Design review of the part built by this model. Coordinates are the model's own, in mm. Face numbers are marked on the shaded views. A direction names the side the tool comes from. Give positions to 0.01 mm unless a question says otherwise; leave off trailing zeros. Loops run counter-clockwise (first coordinate to the right, second up) from the corner with the lowest first, then second, coordinate; pieces in that order, holes last. Notation, with made-up numbers: (79, 87) -> (114, 87) arc R8 cw to (114, 94) -> close; hole circle Ø5 at (2.25, 1.25). An arc over 180 degrees is marked (long way). Answer as CSV lines item,"result".
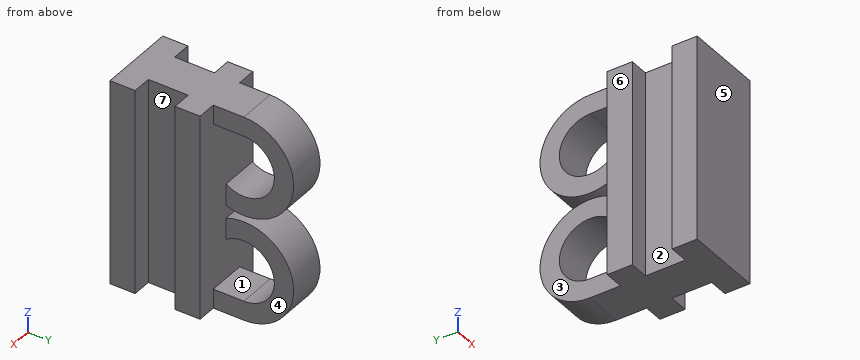
from build123d import *

# Parameters (mm, degrees)
SKETCH1_W           = 15.995688374
SKETCH1_H           = 2
SKETCH1_H_2         = 3
BOSS_EXTRUDE1_DEPTH = 3
SKETCH4_W           = 15.995688374
SKETCH4_H           = 1.95
BOSS_EXTRUDE2_DEPTH = 3


with BuildPart() as part:
    # Sketch1 → Boss-Extrude1 (new body)
    with BuildSketch(Plane(origin=(0, 0, 0), x_dir=(0, 0, -1), z_dir=(1, 0, 0))):
        with BuildLine():
            Line((-7.997844187, 0), (-6.497844187, 0))
            Line((-6.497844187, 0), (-6.497844187, 2.375))
            ThreePointArc((-6.497844187, 2.375), (-3.401228889, 4.637718799), (-2.186352513, 1))
            Line((-2.186352513, 1), (-0.5, 1))
            ThreePointArc((-0.5, 1), (-3.423879317, 6.186439769), (-7.997844187, 2.375))
            Line((-7.997844187, 2.375), (-7.997844187, 0))
        make_face()
        with Locations((0, -1)):
            Rectangle(SKETCH1_W, SKETCH1_H)
        with BuildLine():
            Line((6.497844187, 2.375), (6.497844187, 0))
            Line((6.497844187, 0), (7.997844187, 0))
            Line((7.997844187, 0), (7.997844187, 2.375))
            ThreePointArc((7.997844187, 2.375), (3.423879317, 6.186439769), (0.5, 1))
            Line((0.5, 1), (2.186352513, 1))
            ThreePointArc((2.186352513, 1), (3.401228889, 4.637718799), (6.497844187, 2.375))
        make_face()
        with Locations((0, -3.5)):
            Rectangle(SKETCH1_W, SKETCH1_H_2)
        with Locations((0, -6)):
            Rectangle(SKETCH1_W, SKETCH1_H)
    extrude(amount=BOSS_EXTRUDE1_DEPTH)

    # Sketch4 → Boss-Extrude2 (add, symmetric)
    with BuildSketch(Plane(origin=(1.5, 0, 0), x_dir=(0, 0, -1), z_dir=(1, 0, 0))):
        with Locations((0, -0.975)):
            Rectangle(SKETCH4_W, SKETCH4_H)
        with Locations((0, -6.025)):
            Rectangle(SKETCH4_W, SKETCH4_H)
    extrude(amount=BOSS_EXTRUDE2_DEPTH, both=True)


solid = part.part
Q1. Clearance check with flat-ended pins moving along their axes: pin 1 Ø1.6 at (y, z) = (-4, 1) entering from -X; pin 2 Ø3 at (y, z) = (4.5, -4) entering from +X; pin 3 Ø1.2 at (x, z) = (-1, -2.5) entering from +Y. State where each tip first meets the part, or that it passes through.
Filled sheet:
pin 1,"stops at x = 0"
pin 2,"stops at x = 3"
pin 3,"stops at y = 0"
Q2. We need section C-C, the plane y = 2. State the section outline as (x, z) points.
Filled sheet:
outline,"(0, -8) -> (3, -8) -> (3, -6.5) -> (0, -6.5) -> close; (0, -1.78) -> (3, -1.78) -> (3, -0.27) -> (0, -0.27) -> close; (0, 0.27) -> (3, 0.27) -> (3, 1.78) -> (0, 1.78) -> close; (0, 6.5) -> (3, 6.5) -> (3, 8) -> (0, 8) -> close"
Q3. For the marked faces 1, 2, 3 and 4, list the 3-axis set-ups (+Z, -Z, +X, -X, +Y, -Y) from which the entire face can be reached by the end or side of a thin tool; tool diameter is ignored.
Filled sheet:
face 1,"+X, -X"
face 2,"+Z, -Z, -X"
face 3,"+Z, -Z, -X, +Y"
face 4,"+Z, -Z, +X, +Y"
Q4. We need section D-D, the plane z = 7. State the section outline as (x, y) points, and give its area (3 significant figures).
Filled sheet:
outline,"(-1.5, -7) -> (4.5, -7) -> (4.5, -5.05) -> (3, -5.05) -> (3, -1.95) -> (4.5, -1.95) -> (4.5, 0) -> (3, 0) -> (3, 4.97) -> (0, 4.97) -> (0, 0) -> (-1.5, 0) -> (-1.5, -1.95) -> (0, -1.95) -> (0, -5.05) -> (-1.5, -5.05) -> close"
area,"47.6 mm^2"
Q5. To check wall thickness, follow probe 1 along Y at (x, z) = (-1.1, 5.75); probe 2 along Y at (x, z) = (1.55, 4); probe 3 along X at (y, z) = (-4.25, 0.25). State the ranges of each line that lie inside material, in increasing order. Write a range as from..to.
Filled sheet:
probe 1,"y = -7..-5.05, -1.95..0"
probe 2,"y = -7..0, 4.75..6.25"
probe 3,"x = 0..3"
Q6. We need section A-A, the plane x = 3.9. State the section outline as (y, z) points.
Filled sheet:
outline,"(-7, -8) -> (-5.05, -8) -> (-5.05, 8) -> (-7, 8) -> close; (-1.95, -8) -> (0, -8) -> (0, 8) -> (-1.95, 8) -> close"
Q7. We need section B-B, the plane z = -6.25. State the section outline as (x, y) points.
Filled sheet:
outline,"(-1.5, -7) -> (4.5, -7) -> (4.5, -5.05) -> (3, -5.05) -> (3, -1.95) -> (4.5, -1.95) -> (4.5, 0) -> (-1.5, 0) -> (-1.5, -1.95) -> (0, -1.95) -> (0, -5.05) -> (-1.5, -5.05) -> close; (0, 3.43) -> (3, 3.43) -> (3, 5.61) -> (0, 5.61) -> close"
Q8. The part is to be moulded in two halves that separate along Y. For the marked faces 5, 6 and 7, say which applies: pulls with the +Y half, pulls with the -Y half, needs draft (parallel to the pull), parting line crosses it, or undercut.
Filled sheet:
face 5,"pulls with the -Y half"
face 6,"needs draft"
face 7,"undercut"
